For this review, take the finished solid that the model builds, in its own axes (mm). Coordinates: 2 decimals unless noted, no trailing zeros. Order: outer loops, then holes, each group sorted by start corner. A loop starts at its lowest first (then second) coordinate and runs counter-clockwise, first axis right, second up. Notation, with made-up numbers: (17, -12) - (50, -12) arc R18 ccw to (50, 1) - close; hole circle Ø4 at (64, 19.25). An arc over 180 degrees is marked (long way). One line per item, written item: value. Start each with the question number.
(1) Consider section D-D on x = 20.5. Write out the cut boundary in (y, z).
(2) Consider section B-B on y = -2. Count the separate pieces of the cut face and the enclosed holes in it, then the cut area to 3 significant figures.
(3) To check wall thickness, follow line 1 along Z through (x, y) = (128, -1.85); line 2 along Y through (x, z) = (16, 3.75); line 3 along Y through (x, z) = (89, -2). State the ranges of each line that lie inside material, in increasing order.
(4) Clearance check with flat-ended pins moving along their axes: pin 1 (0.6 mm diameter, centred on x = 57.5, y = 1, fed in from -Z); pin 2 (5 mm diameter, centred on x = 128, z = 0, fed in from +Y). State where each tip first meets the part, or that it passes through.
```python
from build123d import *

# Parameters (mm, degrees)
EXTRUDE_1_DEPTH     = 156
CHAMFER_1_SIZE      = 0.2
CHAMFER_2_SIZE      = 0.1
SKETCH_2_R          = 1.6
CUT_EXTRUDE_1_DEPTH = 6.5
SKETCH_3_R          = 3
CUT_EXTRUDE_2_DEPTH = 3.5


with BuildPart() as part:
    # 草图1 → 凸台-拉伸1 (new body)
    with BuildSketch(Plane(origin=(0, 0, 0), x_dir=(0, 0, -1), z_dir=(1, 0, 0))):
        Polygon((-4.5, 1.5), (-3.5, 1.5), (-3.5, 0.5), (-4.5, 0.5), (-4.5, -3.5), (4.5, -3.5), (4.5, 0.5), (3.5, 0.5), (3.5, 1.5), (4.5, 1.5), (4.5, 3), (-4.5, 3), align=None)
    extrude(amount=EXTRUDE_1_DEPTH)

    # 倒角1
    chamfer_1_edges = [part.edges().sort_by_distance(p)[0] for p in [
        (78, 1.5, -4.5),
        (78, 0.5, -4.5),
        (78, 0.5, 4.5),
        (78, 1.5, 4.5),
        (78, 3, 4.5),
        (78, 3, -4.5),
    ]]
    chamfer(chamfer_1_edges, length=CHAMFER_1_SIZE)

    # 倒角2
    chamfer_2_edges = [part.edges().sort_by_distance(p)[0] for p in [
        (78, 1.5, -3.5),
        (78, 0.5, -3.5),
        (78, -3.5, -4.5),
        (78, -3.5, 4.5),
        (78, 0.5, 3.5),
        (78, 1.5, 3.5),
    ]]
    chamfer(chamfer_2_edges, length=CHAMFER_2_SIZE)

    # 草图2 → 切除-拉伸1 (cut)
    with BuildSketch(Plane(origin=(0, 3, 0), x_dir=(1, 0, 0), z_dir=(0, 1, 0))):
        with Locations(Location((8, 0, 0), (0, 0, 270))):
            Circle(SKETCH_2_R)
        with Locations(Location((28, 0, 0), (0, 0, 270))):
            Circle(SKETCH_2_R)
        with Locations(Location((48, 0, 0), (0, 0, 270))):
            Circle(SKETCH_2_R)
        with Locations(Location((68, 0, 0), (0, 0, 270))):
            Circle(SKETCH_2_R)
        with Locations(Location((88, 0, 0), (0, 0, 270))):
            Circle(SKETCH_2_R)
        with Locations(Location((108, 0, 0), (0, 0, 270))):
            Circle(SKETCH_2_R)
        with Locations(Location((128, 0, 0), (0, 0, 270))):
            Circle(SKETCH_2_R)
        with Locations(Location((148, 0, 0), (0, 0, 270))):
            Circle(SKETCH_2_R)
    extrude(amount=-CUT_EXTRUDE_1_DEPTH, mode=Mode.SUBTRACT)

    # 草图3 → 切除-拉伸2 (cut)
    with BuildSketch(Plane(origin=(0, 3, 0), x_dir=(1, 0, 0), z_dir=(0, 1, 0))):
        with Locations(Location((8, 0, 0), (0, 0, 270))):
            Circle(SKETCH_3_R)
        with Locations(Location((28, 0, 0), (0, 0, 270))):
            Circle(SKETCH_3_R)
        with Locations(Location((48, 0, 0), (0, 0, 270))):
            Circle(SKETCH_3_R)
        with Locations(Location((68, 0, 0), (0, 0, 270))):
            Circle(SKETCH_3_R)
        with Locations(Location((88, 0, 0), (0, 0, 270))):
            Circle(SKETCH_3_R)
        with Locations(Location((108, 0, 0), (0, 0, 270))):
            Circle(SKETCH_3_R)
        with Locations(Location((128, 0, 0), (0, 0, 270))):
            Circle(SKETCH_3_R)
        with Locations(Location((148, 0, 0), (0, 0, 270))):
            Circle(SKETCH_3_R)
    extrude(amount=-CUT_EXTRUDE_2_DEPTH, mode=Mode.SUBTRACT)


solid = part.part
```
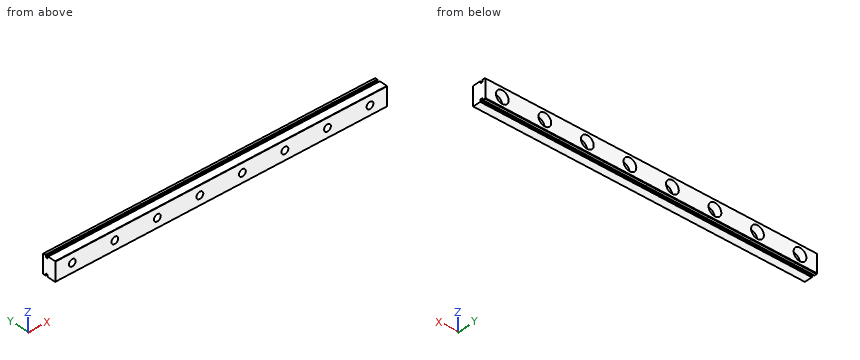
Geometry check:
1. outline: (-3.5, -4.4) - (-3.4, -4.5) - (0.3, -4.5) - (0.5, -4.3) - (0.5, -3.6) - (0.6, -3.5) - (1.4, -3.5) - (1.5, -3.6) - (1.5, -4.3) - (1.7, -4.5) - (2.8, -4.5) - (3, -4.3) - (3, 4.3) - (2.8, 4.5) - (1.7, 4.5) - (1.5, 4.3) - (1.5, 3.6) - (1.4, 3.5) - (0.6, 3.5) - (0.5, 3.6) - (0.5, 4.3) - (0.3, 4.5) - (-3.4, 4.5) - (-3.5, 4.4) - close
2. separate pieces: 1
2. enclosed holes: 8
2. area: 1,340 mm^2
3. line 1: z = -4.5 to -1.6, 1.6 to 4.5
3. line 2: y = -3.5 to 0.5, 1.5 to 3
3. line 3: y = -3.5 to -0.5
4. pin 1: stops at z = -3.5
4. pin 2: stops at y = -0.5
